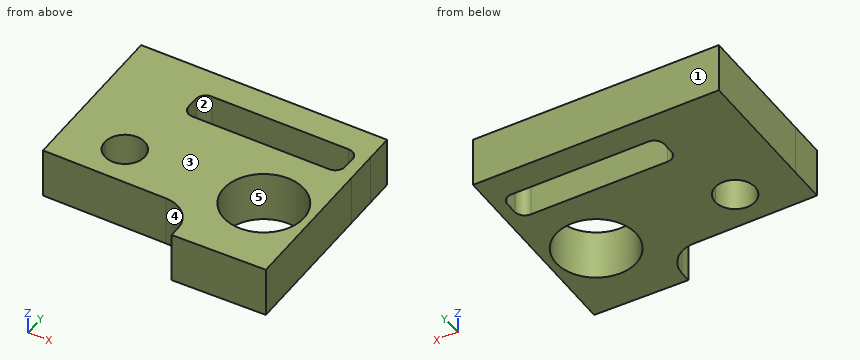
```python
from build123d import *

# Parameters (mm, degrees)
F0_R     = 20
F1_DEPTH = 25


with BuildPart() as f1:
    # F0 (on Top) → F1 (new body)
    with BuildSketch(Plane.XY):
        with BuildLine():
            ThreePointArc((-60.707048, -16.170189), (-70.798248, -6.170605), (-80.705385, -16.352581))
            ThreePointArc((-80.705385, -16.352581), (-70.615848, -26.169773), (-60.707048, -16.170189))
        make_face()
        with BuildLine():
            Line((17.155273, 48.271821), (-101.887608, 48.271821))
            Line((-101.887608, 48.271821), (-100.702058, -16.717366))
            Line((-100.702058, -16.717366), (-100.365747, -35.153195))
            Line((-100.365747, -35.153195), (-38.009589, -35.493795))
            ThreePointArc((-38.009589, -35.493795), (-27.553158, -39.819167), (-23.094029, -50.219261))
            Line((-23.094029, -50.219261), (-22.996154, -55.570459))
            Line((-22.996154, -55.570459), (23.995987, -54.710954))
            Line((23.995987, -54.710954), (22.661012, 18.276838))
            Line((22.661012, 18.276838), (22.368415, 34.274162))
            Line((22.368415, 34.274162), (22.112392, 48.271821))
            Line((22.112392, 48.271821), (17.155273, 48.271821))
        make_face()
        with BuildLine():
            ThreePointArc((-60.707048, -16.170189), (-70.615848, -26.169773), (-80.705385, -16.352581))
            ThreePointArc((-80.705385, -16.352581), (-70.798248, -6.170605), (-60.707048, -16.170189))
        make_face(mode=Mode.SUBTRACT)
        with Locations((-0.478208, -16.36657)):
            Circle(F0_R, mode=Mode.SUBTRACT)
        with BuildLine():
            ThreePointArc((11.401503, 34.126978), (14.937037, 32.662512), (16.401503, 29.126978))
            Line((16.401503, 29.126978), (16.401503, 23.126978))
            ThreePointArc((16.401503, 23.126978), (14.937037, 19.591444), (11.401503, 18.126978))
            Line((11.401503, 18.126978), (-57.598497, 18.126978))
            ThreePointArc((-57.598497, 18.126978), (-61.134031, 19.591444), (-62.598497, 23.126978))
            Line((-62.598497, 23.126978), (-62.598497, 29.126978))
            ThreePointArc((-62.598497, 29.126978), (-61.134031, 32.662512), (-57.598497, 34.126978))
            Line((-57.598497, 34.126978), (11.401503, 34.126978))
        make_face(mode=Mode.SUBTRACT)
    extrude(amount=F1_DEPTH)


solid = f1.part
```
Build history of the part. All positions in model axes, mm. Face numbers are marked on the shaded views. A direction names the side the tool comes from. Round coordinates to 2 decimals unless told otherwise and drop trailing zeros. Write each loop counter-clockwise with the first axis right and the second up, starting at its lowest first coordinate (ties: lowest second). Pieces come first, ordered by that corner, then holes. Notation, with made-up numbers: (54, 39) -> (112, 39) arc R22 cw to (112, 54) -> close; hole circle Ø5 at (-20.5, 23.25). An arc over 180 degrees is marked (long way). Put each result on its own line as item: value.
Item 1: Wall check: probe 1 along Y at (x, z) = (-18, 10); probe 2 along X at (y, z) = (-9, 8.5); probe 3 along Y at (x, z) = (6, 4.75). Give the ranges that are in metal, low to high. Write a range as from..to.
Here are the results:
probe 1: y = -55.48..-26.01, -6.72..18.13, 34.13..48.27
probe 2: x = -100.84..-77.68, -63.74..-19.07, 18.12..23.16
probe 3: y = -55.04..-35.29, 2.56..18.13, 34.13..48.27
Item 2: Slice it at A-A, the plane x = -0.5. Give the cut face in (y, z).
Here are the results:
outline: (-55.16, 0) -> (-36.37, 0) -> (-36.37, 25) -> (-55.16, 25) -> close; (3.63, 0) -> (18.13, 0) -> (18.13, 25) -> (3.63, 25) -> close; (34.13, 0) -> (48.27, 0) -> (48.27, 25) -> (34.13, 25) -> close
Item 3: Slice it at C-C, the plane y = -1. Give the cut face in (x, z), plus the area to 3 significant figures.
Here are the results:
outline: (-100.99, 0) -> (-13.28, 0) -> (-13.28, 25) -> (-100.99, 25) -> close; (12.32, 0) -> (23.01, 0) -> (23.01, 25) -> (12.32, 25) -> close
area: 2,460 mm^2
Item 4: Tool access for the marked faces 1 and 2: list every direction of +Z, -Z, +X, -X, +Y, -Y with a clear straight run to the whole face (end or side of a thin tool).
Here are the results:
face 1: +Z, -Z, +X, -X, +Y
face 2: +Z, -Z
Item 5: Two-plate mould, pull along X, no slides. Class the marked faces 3, 4 and 5: pulls with the +X half, pulls with the -X half, needs draft (parallel to the pull), parting line crosses it, or undercut.
Here are the results:
face 3: needs draft
face 4: pulls with the -X half
face 5: undercut
Item 6: Slice it at D-D, the plane x = -54. Give the cut face in (y, z), plus the area to 3 significant figures.
Here are the results:
outline: (-35.41, 0) -> (18.13, 0) -> (18.13, 25) -> (-35.41, 25) -> close; (34.13, 0) -> (48.27, 0) -> (48.27, 25) -> (34.13, 25) -> close
area: 1,690 mm^2
Item 7: Slice it at B-B, the plane z = 15.75. Give the cut face in (x, y).
Here are the results:
outline: (-101.89, 48.27) -> (-100.37, -35.15) -> (-38.01, -35.49) arc R15 cw to (-23.09, -50.22) -> (-23, -55.57) -> (24, -54.71) -> (22.11, 48.27) -> close; hole circle Ø20 at (-70.71, -16.17); hole (-62.6, 23.13) arc R5 ccw to (-57.6, 18.13) -> (11.4, 18.13) arc R5 ccw to (16.4, 23.13) -> (16.4, 29.13) arc R5 ccw to (11.4, 34.13) -> (-57.6, 34.13) arc R5 ccw to (-62.6, 29.13) -> close; hole circle Ø40 at (-0.48, -16.37)
Item 8: Flat gauge pins, fed straight in: P1, Ø3, axis at y = 25.5, z = 17.5, coming from the -X side; P2, Ø12, axis at x = -1.5, z = 21, coming from the -Y side; P3, Ø3, axis at y = 24.5, z = 16.5, coming from the +X side. Where does each tip first touch, or does it go through?
Here are the results:
P1: stops at x = -101.5
P2: stops at y = -55.29
P3: stops at x = 22.57
